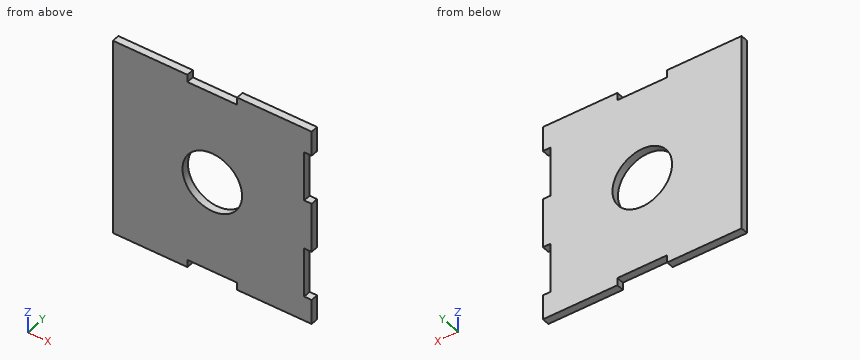
```python
from build123d import *

# Parameters (mm, degrees)
CROQUIS1_R              = 12
SALIENTE_EXTRUIR1_DEPTH = 3


with BuildPart() as part:
    # Croquis1 → Saliente-Extruir1 (new body)
    with BuildSketch(Plane(origin=(0, 0, 0), x_dir=(1, 0, 0), z_dir=(0, 1, 0))):
        Polygon((-40, 40), (-10, 40), (-10, 37), (0, 37), (10, 37), (10, 40), (37, 40), (40, 40), (40, 30), (37, 30), (37, 10), (40, 10), (40, -10), (37, -10), (37, -30), (40, -30), (40, -40), (37, -40), (10, -40), (10, -37), (0, -37), (-10, -37), (-10, -40), (-40, -40), align=None)
        with Locations(Location((0, 0, 0), (0, 0, 270))):
            Circle(CROQUIS1_R, mode=Mode.SUBTRACT)
    extrude(amount=SALIENTE_EXTRUIR1_DEPTH)


solid = part.part
```
Could you check a few things on this model? Use its own coordinates, in mm. Round coordinates to 2 decimals unless told otherwise and drop trailing zeros. Write each loop counter-clockwise with the first axis right and the second up, starting at its lowest first coordinate (ties: lowest second). Pieces come first, ordered by that corner, then holes. Notation, with made-up numbers: M 73,68.5 L 126,68.5 A28 ccw 126,89.5 Z; hole C 52.25,75.5 d7. An arc over 180 degrees is marked long. Answer in a Markdown table with one row per item. Add a question column.
Q1. Will these pins go through, and if not, where does the flat tip stop? pin 1 Ø0.9 at (y, z) = (1, 23) entering from +X; pin 2 Ø1.5 at (x, y) = (-2.5, 1.5) entering from -Z; pin 3 Ø1.5 at (x, y) = (-1.5, 1.5) entering from +Z.
Q2. If I drill on line 1 (X direction, y = 1, z = 0); line 2 (X direction, y = 2.25, z = -18.5); line 3 (Z direction, x = -1.5, y = 0.65), over which ranges is the centre line in solid material (lowest first)? Write a range as from..to.
Q3. Imagine slicing it at B-B (z = 0). Please give me the cut outline in (x, y).
Q4. Imagine slicing it at C-C (z = 13). Please give me the cut outline in (x, y), then the cut area to 3 significant figures.
Q5. Imagine slicing it at A-A (x = 0). Please give me the cut outline in (y, z).
Values:
| question | item | result |
|---|---|---|
| 1 | pin 1 | x = 37 |
| 1 | pin 2 | z = -37 |
| 1 | pin 3 | z = 37 |
| 2 | line 1 | -40..-12, 12..40 |
| 2 | line 2 | -40..37 |
| 2 | line 3 | -37..-11.91, 11.91..37 |
| 3 | outline | M -40,0 L -12,0 L -12,3 L -40,3 Z; M 12,0 L 40,0 L 40,3 L 12,3 Z |
| 4 | outline | M -40,0 L 37,0 L 37,3 L -40,3 Z |
| 4 | area | 231 mm^2 |
| 5 | outline | M 0,-37 L 3,-37 L 3,-12 L 0,-12 Z; M 0,12 L 3,12 L 3,37 L 0,37 Z |
